from build123d import *

# Parameters (mm, degrees)
ESQUISSE1_R             = 363.2
BOSS_EXTRU_1_DEPTH      = 10
ESQUISSE2_R             = 143.2
BOSS_EXTRU_2_DEPTH      = 100
ESQUISSE4_W             = 5
ESQUISSE4_H             = 220
ENL_V_MAT_EXTRU_1_DEPTH = 524.286231426


with BuildPart() as part:
    # Esquisse1 → Boss.-Extru.1 (new body)
    with BuildSketch(Plane.XY):
        Circle(ESQUISSE1_R)
    extrude(amount=BOSS_EXTRU_1_DEPTH)

    # Esquisse2 → Boss.-Extru.2 (add)
    with BuildSketch(Plane.XY.offset(10)):
        Circle(ESQUISSE2_R)
    extrude(amount=BOSS_EXTRU_2_DEPTH)

    # Esquisse4 → Enlèv. mat.-Extru.1 (cut, through all)
    with BuildSketch(Plane.XY.offset(10)):
        with Locations((0, -253.1)):
            Rectangle(ESQUISSE4_W, ESQUISSE4_H)
    extrude(amount=-ENL_V_MAT_EXTRU_1_DEPTH, mode=Mode.SUBTRACT)


solid = part.part
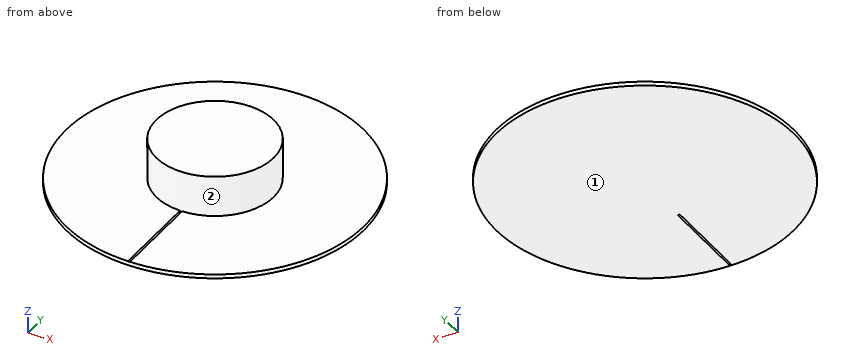
Build history of the part. All positions in model axes, mm. Face numbers are marked on the shaded views. A direction names the side the tool comes from. Round coordinates to 2 decimals unless told otherwise and drop trailing zeros. Write each loop counter-clockwise with the first axis right and the second up, starting at its lowest first coordinate (ties: lowest second). Pieces come first, ordered by that corner, then holes. Notation, with made-up numbers: M 11,-39 L 58,-39 A22 ccw 58,-8 Z; hole C -34.75,60.5 d9. An arc over 180 degrees is marked long. Answer as a JSON object with one key per item and string values. Group by question number.
(1) Which spindle directions (+Z, -Z, +X, -X, +Y, -Y) get a long thin tool onto all of the face, cutting with end or side? Do the marked faces 1 and 2. Say none if no direction does.
(2) Cut at C-C (x = 74). Give the cut face in (y, z), and give its area (3 significant figures).
(3) Drill centre lines: L1, parallel to Z at x = 251, y = -260.5; L2, parallel to Y at x = -106.5, z = 11.5; L3, parallel to X at y = -114, z = 51.5. Where is each one in solid material? Low to high.
(4) Cut at B-B (y = -195.5). Give the cut face in (x, z), and give its area (3 significant figures).
(5) Flat gauge pins, fed straight in: pin 1 (3 mm diameter, centred on x = -105, z = 54, fed in from +Y); pin 2 (2 mm diameter, centred on x = 112.5, y = -205.5, fed in from +Z); pin 3 (8 mm diameter, centred on y = -240.5, z = 5.5, fed in from -X). Where does each tip first touch, or does it go through?
(6) Cut at D-D (z = 32.5). Give the cut face in (x, y), and give its area (3 significant figures).
(7) Cut at A-A (y = 0). Give the cut face in (x, z), and give its area (3 significant figures).
Responses:
{
 "1": {"face 1": "-Z, +X, -X, +Y, -Y", "face 2": "+Z"},
 "2": {"outline": "M -355.58,0 L 355.58,0 L 355.58,10 L 122.6,10 L 122.6,110 L -122.6,110 L -122.6,10 L -355.58,10 Z", "area": "31,600 mm2"},
 "3": {"L1": "z = 0 to 10", "L2": "y = -95.73 to 95.73", "L3": "x = -86.66 to 86.66"},
 "4": {"outline": "M -306.09,0 L -2.5,0 L -2.5,10 L -306.09,10 Z; M 2.5,0 L 306.09,0 L 306.09,10 L 2.5,10 Z", "area": "6,070 mm2"},
 "5": {"pin 1": "stops at y = 98.96", "pin 2": "stops at z = 10", "pin 3": "stops at x = -275.65"},
 "6": {"outline": "C 0,0 d286.4", "area": "64,400 mm2"},
 "7": {"outline": "M -363.2,0 L 363.2,0 L 363.2,10 L 143.2,10 L 143.2,110 L -143.2,110 L -143.2,10 L -363.2,10 Z", "area": "35,900 mm2"}
}
